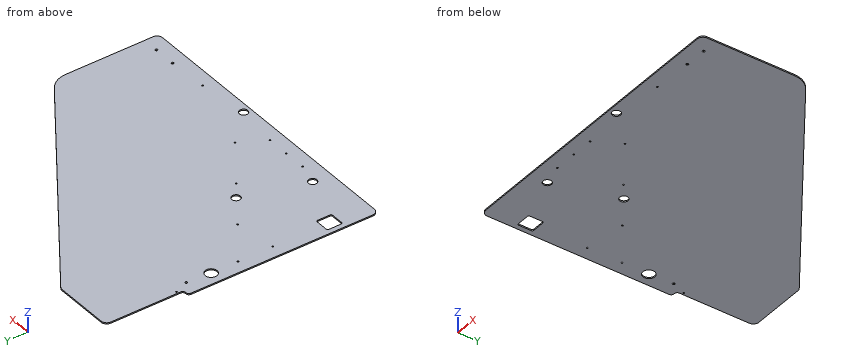
from build123d import *

# Parameters (mm, degrees)
SKETCH1_R           = 19.05
SKETCH1_R_2         = 26.987499999
SKETCH1_R_3         = 3.556
SKETCH1_R_4         = 5.55625
SKETCH1_R_5         = 3.175
SKETCH1_R_6         = 5.3578125
BOSS_EXTRUDE1_DEPTH = 5.588


with BuildPart() as part:
    # Sketch1 → Boss-Extrude1 (new body)
    with BuildSketch(Plane.XY):
        with BuildLine():
            Line((1368.43262, 25.4), (1368.43262, 421.546809256))
            ThreePointArc((1368.43262, 421.546809256), (1356.952920651, 468.460468361), (1325.107985933, 504.772656956))
            Line((1325.107985933, 504.772656956), (311.360252246, 1214.606461927))
            ThreePointArc((311.360252246, 1214.606461927), (304.42933807, 1218.024410551), (296.791410762, 1219.200000002))
            Line((296.791410762, 1219.200000002), (53.975, 1219.200000002))
            ThreePointArc((53.975, 1219.200000002), (36.014487758, 1211.760512244), (28.575, 1193.800000002))
            Line((28.575, 1193.800000002), (28.575, 876.300000002))
            ThreePointArc((28.575, 876.300000002), (24.855256121, 867.319743881), (15.875, 863.600000002))
            Line((15.875, 863.600000002), (12.7, 863.600000002))
            ThreePointArc((12.7, 863.600000002), (3.719743879, 859.880256123), (0, 850.900000002))
            Line((0, 850.900000002), (0, 25.4))
            ThreePointArc((0, 25.4), (7.439487758, 7.439487758), (25.4, 0))
            Line((25.4, 0), (1343.03262, 0))
            ThreePointArc((1343.03262, 0), (1360.993132242, 7.439487758), (1368.43262, 25.4))
        make_face()
        with Locations((794.6898, 32.562800001)):
            Circle(SKETCH1_R, mode=Mode.SUBTRACT)
        with Locations((381.27686, 367.8301)):
            Circle(SKETCH1_R, mode=Mode.SUBTRACT)
        with Locations((57.150106704, 717.550000002)):
            Circle(SKETCH1_R_2, mode=Mode.SUBTRACT)
        with Locations((297.48226, 81.5975)):
            Circle(SKETCH1_R, mode=Mode.SUBTRACT)
        with Locations((57.150106704, 595.973055669)):
            Circle(SKETCH1_R_3, mode=Mode.SUBTRACT)
        with Locations((57.150106704, 438.150000002)):
            Circle(SKETCH1_R_3, mode=Mode.SUBTRACT)
        with Locations((243.943004281, 461.107910727)):
            Circle(SKETCH1_R_3, mode=Mode.SUBTRACT)
        with Locations((452.007623531, 315.419495894)):
            Circle(SKETCH1_R_3, mode=Mode.SUBTRACT)
        with Locations((660.07224278, 169.731081062)):
            Circle(SKETCH1_R_3, mode=Mode.SUBTRACT)
        with Locations((393.7, 57.150000001)):
            Circle(SKETCH1_R_3, mode=Mode.SUBTRACT)
        with Locations((495.3, 57.150000001)):
            Circle(SKETCH1_R_3, mode=Mode.SUBTRACT)
        with Locations((596.9, 57.150000001)):
            Circle(SKETCH1_R_3, mode=Mode.SUBTRACT)
        with Locations((1016, 57.150000001)):
            Circle(SKETCH1_R_3, mode=Mode.SUBTRACT)
        with Locations((1193.80762, 63.5)):
            Circle(SKETCH1_R_4, mode=Mode.SUBTRACT)
        with Locations((1295.40762, 63.5)):
            Circle(SKETCH1_R_4, mode=Mode.SUBTRACT)
        with Locations((38.1, 889.000000002)):
            Circle(SKETCH1_R_5, mode=Mode.SUBTRACT)
        with Locations((63.5, 825.500000002)):
            Circle(SKETCH1_R_6, mode=Mode.SUBTRACT)
        with BuildLine():
            Line((22.225, 209.550000002), (22.225, 152.400000002))
            ThreePointArc((22.225, 152.400000002), (24.084871939, 147.909871941), (28.575, 146.050000002))
            Line((28.575, 146.050000002), (85.725, 146.050000002))
            ThreePointArc((85.725, 146.050000002), (90.215128061, 147.909871941), (92.075, 152.400000002))
            Line((92.075, 152.400000002), (92.075, 209.550000002))
            ThreePointArc((92.075, 209.550000002), (90.215128061, 214.040128062), (85.725, 215.900000002))
            Line((85.725, 215.900000002), (28.575, 215.900000002))
            ThreePointArc((28.575, 215.900000002), (24.084871939, 214.040128062), (22.225, 209.550000002))
        make_face(mode=Mode.SUBTRACT)
    extrude(amount=BOSS_EXTRUDE1_DEPTH)


solid = part.part
Source: CAD feature listing. Evaluate the final solid. Frame: model axes, mm. Give positions to 0.01 mm unless a question says otherwise; leave off trailing zeros. Order: outer loops, then holes, each group sorted by start corner. A loop starts at its lowest first (then second) coordinate and runs counter-clockwise, first axis right, second up. Notation, with made-up numbers: (-1, -35.5) -> (56, -35.5) arc R18 cw to (56, -13.5) -> close; hole circle Ø3 at (75, 20). An arc over 180 degrees is marked (long way). Use a Markdown table: item, result.
1) Contact query for a flat-ended pin moving along its axis: P1, Ø1.5, axis at x = 1133, z = 4, coming from the +Y side. Output: stop coordinate, or through.
Answer list:
| item | result |
|---|---|
| P1 | y = 639.81 |
2) Section query A-A, the plane x = 1260.5. Return the cut outline in (y, z).
Answer list:
| item | result |
|---|---|
| outline | (0, 0) -> (550.01, 0) -> (550.01, 5.59) -> (0, 5.59) -> close |
3) Section query B-B, the plane y = 948.5. Return the cut outline in (x, z) (3 decimals), then the cut area to 3 significant figures.
Answer list:
| item | result |
|---|---|
| outline | (28.575, 0) -> (691.4, 0) -> (691.4, 5.588) -> (28.575, 5.588) -> close |
| area | 3,700 mm² |
4) Ray query, line 1 along X through (y, z) = (168.5, 1.6) (3 decimals); line 2 along X through (y, z) = (720.5, 1.55); line 3 along Y through (x, z) = (306, 2.75). Return the intervals inside material, ascending. Write a range as [from, to].
Answer list:
| item | result |
|---|---|
| line 1 | [0, 22.225], [92.075, 656.736], [663.408, 1368.433] |
| line 2 | [0, 30.32], [83.98, 1017.02] |
| line 3 | [0, 64.56], [98.64, 1217.47] |
